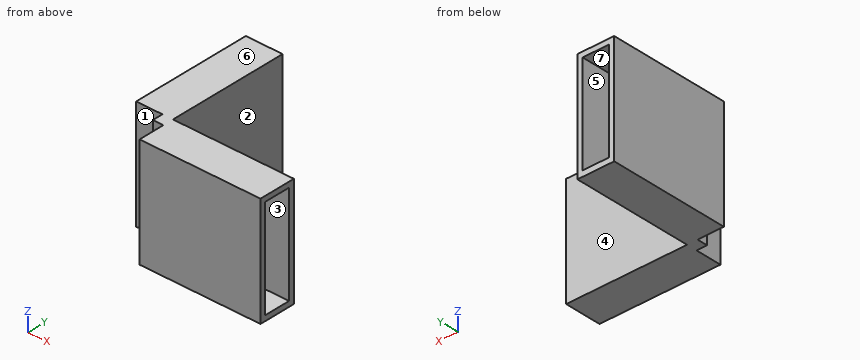
from build123d import *

# Parameters (mm, degrees)
SKETCH1_W           = 30
SKETCH1_H           = 30
BOSS_EXTRUDE1_DEPTH = 7
SKETCH2_W           = 7
SKETCH2_H           = 23
BOSS_EXTRUDE4_DEPTH = 20
SKETCH4_W           = 2
SKETCH4_H           = 2
BOSS_EXTRUDE6_DEPTH = 20
SKETCH5_W           = 23
SKETCH5_H           = 7
BOSS_EXTRUDE7_DEPTH = 20
SHELL2_START        = 8
SHELL2_DEPTH        = 22
SHELL2_START_2      = 1
SHELL2_2_DEPTH      = 5
SHELL2_START_3      = 6
SHELL2_3_OUTLINE_W  = 29
SHELL2_3_OUTLINE_H  = 5
SHELL2_3_DEPTH      = 2
SKETCH7_W           = 23
SKETCH7_H           = 1
BOSS_EXTRUDE8_DEPTH = 5
SKETCH9_W           = 1.075143629
SKETCH9_H           = 23
BOSS_EXTRUDE9_DEPTH = 5
SKETCH10_W          = 30
SKETCH10_H          = 30
CUT_EXTRUDE1_DEPTH  = 6
CUT_EXTRUDE2_DEPTH  = 6
SKETCH12_W          = 23
SKETCH12_H          = 23
CUT_EXTRUDE3_DEPTH  = 6


# Read off the part's stored shape, not the designer's step: Shell2
with BuildPart() as part:
    # Sketch1 → Boss-Extrude1 (new body)
    with BuildSketch(Plane.XY):
        with Locations((15, 15)):
            Rectangle(SKETCH1_W, SKETCH1_H)
    extrude(amount=BOSS_EXTRUDE1_DEPTH)

    # Sketch2 → Boss-Extrude4 (add)
    with BuildSketch(Plane.XY.offset(7)):
        with Locations((3.5, 18.5)):
            Rectangle(SKETCH2_W, SKETCH2_H)
    extrude(amount=BOSS_EXTRUDE4_DEPTH)

    # Sketch4 → Boss-Extrude6 (add)
    with BuildSketch(Plane.XY.offset(7)):
        with Locations((6, 6)):
            Rectangle(SKETCH4_W, SKETCH4_H)
    extrude(amount=BOSS_EXTRUDE6_DEPTH)

    # Sketch5 → Boss-Extrude7 (add)
    with BuildSketch(Plane.XY.offset(7)):
        with Locations((18.5, 3.5)):
            Rectangle(SKETCH5_W, SKETCH5_H)
    extrude(amount=BOSS_EXTRUDE7_DEPTH)

    # Shell2 outline → Shell2 (cut)
    with BuildSketch(Plane(origin=(0, 0, 0), x_dir=(1, 0, 0), z_dir=(0, 1, 0)).offset(SHELL2_START)):
        Polygon((6, -6), (30, -6), (30, -1), (1, -1), (1, -26), (6, -26), align=None)
    extrude(amount=SHELL2_DEPTH, mode=Mode.SUBTRACT)

    # Shell2 2 outline → Shell2 2 (cut)
    with BuildSketch(Plane(origin=(0, 0, 0), x_dir=(1, 0, 0), z_dir=(0, 1, 0)).offset(SHELL2_START_2)):
        Polygon((8, -6), (8, -26), (30, -26), (30, -1), (1, -1), (1, -6), align=None)
    extrude(amount=SHELL2_2_DEPTH, mode=Mode.SUBTRACT)

    # Shell2 3 outline → Shell2 3 (cut)
    with BuildSketch(Plane(origin=(0, 0, 0), x_dir=(1, 0, 0), z_dir=(0, 1, 0)).offset(SHELL2_START_3)):
        with Locations((15.5, -3.5)):
            Rectangle(SHELL2_3_OUTLINE_W, SHELL2_3_OUTLINE_H)
    extrude(amount=SHELL2_3_DEPTH, mode=Mode.SUBTRACT)

    # Sketch7 → Boss-Extrude8 (add)
    with BuildSketch(Plane.XZ.offset(-6)):
        with Locations((18.5, 6.5)):
            Rectangle(SKETCH7_W, SKETCH7_H)
    extrude(amount=BOSS_EXTRUDE8_DEPTH)

    # Sketch9 → Boss-Extrude9 (add)
    with BuildSketch(Plane.ZY.offset(-6)):
        with Locations((6.537571814, 18.5)):
            Rectangle(SKETCH9_W, SKETCH9_H)
    extrude(amount=BOSS_EXTRUDE9_DEPTH)

    # Sketch10 → Cut-Extrude1 (cut)
    with BuildSketch(Plane(origin=(0, 0, 0), x_dir=(-1, 0, 0), z_dir=(0, 0, -1))):
        with Locations((-15, 15)):
            Rectangle(SKETCH10_W, SKETCH10_H)
    extrude(amount=-CUT_EXTRUDE1_DEPTH, mode=Mode.SUBTRACT)

    # Sketch11 → Cut-Extrude2 (cut)
    with BuildSketch(Plane.XY.offset(7)):
        Polygon((7, 0), (7, 5), (5, 5), (5, 7), (0, 7), (0, 0), align=None)
    extrude(amount=-CUT_EXTRUDE2_DEPTH, mode=Mode.SUBTRACT)

    # Sketch12 → Cut-Extrude3 (cut)
    with BuildSketch(Plane.XY.offset(7)):
        with Locations((18.5, 18.5)):
            Rectangle(SKETCH12_W, SKETCH12_H)
    extrude(amount=-CUT_EXTRUDE3_DEPTH, mode=Mode.SUBTRACT)


solid = part.part
The model under review builds one solid part; all positions refer to its coordinate system, in mm. Face numbers are marked on the shaded views. A direction names the side the tool comes from. Coordinates: 2 decimals unless noted, no trailing zeros. Loops run counter-clockwise (first coordinate to the right, second up) from the corner with the lowest first, then second, coordinate; pieces in that order, holes last.
(1) Consider section B-B, the plane y = 22.25. Give the boundary of the cut face in (x, z).
Determined:
outline: (0, 6) - (7, 6) - (7, 27) - (0, 27) - close; hole (1, 7.08) - (6, 7.08) - (6, 26) - (1, 26) - close
(2) Consider section D-D, the plane x = 3. Give the boundary of the cut face in (y, z), plus the area to 3 significant figures.
Determined:
outline: (7, 6) - (30, 6) - (30, 7.08) - (8, 7.08) - (8, 26) - (30, 26) - (30, 27) - (7, 27) - close
area: 66.7 mm2
(3) Wall thickness on L1, parallel to Y at x = 8.75, z = 20.5; L2, parallel to Z at x = 3.5, y = 22; L3, parallel to Z at x = 18, y = 4: over which ranges is each line inside the solid? List them lowest first.
Determined:
L1: y = 0 to 1, 6 to 7
L2: z = 6 to 7.08, 26 to 27
L3: z = 6 to 7, 26 to 27
(4) Insertion check: P1, Ø0.6, axis at y = 6, z = 15, coming from the -X side; P2, Ø1, axis at x = 27, z = 13.5, coming from the +Y side; P3, Ø4, axis at y = 1.5, z = 20.5, coming from the -X side. Each pin has a flat end and moves straight along its axis. Give the tip position at first contact, or say it passes through.
Determined:
P1: stops at x = 5
P2: stops at y = 7
P3: stops at x = 7
(5) Consider section C-C, the plane z = 22.25. Give the boundary of the cut face in (x, y), plus the area to 3 significant figures.
Determined:
outline: (0, 7) - (5, 7) - (5, 5) - (7, 5) - (7, 0) - (30, 0) - (30, 1) - (8, 1) - (8, 6) - (30, 6) - (30, 7) - (7, 7) - (7, 30) - (6, 30) - (6, 8) - (1, 8) - (1, 30) - (0, 30) - close
area: 106 mm2
(6) Tool access review of the marked faces 1, 2 and 3: name each direction out of +Z, -Z, +X, -X, +Y, -Y from which nothing blocks a thin tool from reaching the whole face with its end or side.
Determined:
face 1: +Z, -Z, -X, -Y
face 2: +Z, -Z, +X, +Y
face 3: +X
(7) Consider section A-A, the plane x = 26.25. Give the boundary of the cut face in (y, z), plus the area to 3 significant figures.
Determined:
outline: (0, 6) - (7, 6) - (7, 27) - (0, 27) - close; hole (1, 7) - (6, 7) - (6, 26) - (1, 26) - close
area: 52.0 mm2
(8) Draft analysis for pull direction Z (two halves, no side actions). For the marked faces 4, 5, 6 and 7, state which applies: +Z half, -Z half, draft (parallel to the pull), parting line (faces both ways), or undercut.
Determined:
face 4: draft
face 5: undercut
face 6: +Z half
face 7: undercut
